```python
from build123d import *

# Parameters (mm, degrees)
SKETCH_R      = 1.75
EXTRUDE_DEPTH = 1


with BuildPart() as part:
    # Sketch → Extrude (new body)
    with BuildSketch(Plane.XY):
        with BuildLine():
            Line((65.264214, 54.65), (67.4, 52.514214))
            Line((67.4, 52.514214), (67.4, 41.014214))
            Line((67.4, 41.014214), (69.95, 38.464214))
            Line((69.95, 38.464214), (69.95, 4.685786))
            Line((69.95, 4.685786), (67.4, 2.135786))
            Line((67.4, 2.135786), (67.4, 1))
            ThreePointArc((65.4, -1), (66.814214, -0.414214), (67.4, 1))
            Line((65.4, -1), (1, -1))
            ThreePointArc((-1, 1), (-0.414214, -0.414214), (1, -1))
            Line((-1, 1), (-1, 52.65))
            ThreePointArc((1, 54.65), (-0.414214, 54.064214), (-1, 52.65))
            Line((1, 54.65), (65.264214, 54.65))
        make_face()
        with Locations((14.05247, 2.556984)):
            Circle(SKETCH_R, mode=Mode.SUBTRACT)
        with Locations((66.413926, 7.668398)):
            Circle(SKETCH_R, mode=Mode.SUBTRACT)
        with Locations((66.409951, 35.749834)):
            Circle(SKETCH_R, mode=Mode.SUBTRACT)
        with Locations((15.334135, 51.082933)):
            Circle(SKETCH_R, mode=Mode.SUBTRACT)
    extrude(amount=EXTRUDE_DEPTH)


solid = part.part
```
Source: CAD feature listing. Evaluate the final solid. Frame: model axes, mm. Give positions to 0.01 mm unless a question says otherwise; leave off trailing zeros. Loops run counter-clockwise (first coordinate to the right, second up) from the corner with the lowest first, then second, coordinate; pieces in that order, holes last. Notation, with made-up numbers: (-6, 68.25) -> (41, 68.25) arc R32 ccw to (41, 100.25) -> close; hole circle Ø7 at (-39.5, 21.25). An arc over 180 degrees is marked (long way). Use a Markdown table: item, result. Add a question column.
(1) Section query B-B (y = 42). Output: boundary loops of the cut face in (x, z), then the cut area to 3 significant figures.
(2) Ray query, line 1 (Y direction, x = 15, z = 0.45); line 2 (Y direction, x = 65, z = 0.55); line 3 (X direction, y = 43, z = 0.5). Return the intervals inside material, ascending.
(3) Pull-direction query (X, two-part tool) for faces 1 (the face through (-0.43, -0.4, 0.49)), 2 (the face through (68.693, 3.429, 0.493)), 3 (the face through (35, 27, 0)), 4 (the face through (68.083, 8.194, 0.493)); classes: +X half, -X half, draft (parallel to the pull), parting line (faces both ways), or undercut.
(4) Section query A-A (z = 0.8). Output: boundary loops of the cut face in (x, y), then the cut area to 3 significant figures.
Checked values:
| question | item | result |
|---|---|---|
| 1 | outline | (-1, 0) -> (67.4, 0) -> (67.4, 1) -> (-1, 1) -> close |
| 1 | area | 68.4 mm^2 |
| 2 | line 1 | -1 to 1.09, 4.03 to 49.37, 52.8 to 54.65 |
| 2 | line 2 | -1 to 6.64, 8.7 to 34.71, 36.79 to 54.65 |
| 2 | line 3 | -1 to 67.4 |
| 3 | face 1 | -X half |
| 3 | face 2 | +X half |
| 3 | face 3 | draft |
| 3 | face 4 | undercut |
| 4 | outline | (-1, 1) arc R2 ccw to (1, -1) -> (65.4, -1) arc R2 ccw to (67.4, 1) -> (67.4, 2.14) -> (69.95, 4.69) -> (69.95, 38.46) -> (67.4, 41.01) -> (67.4, 52.51) -> (65.26, 54.65) -> (1, 54.65) arc R2 ccw to (-1, 52.65) -> close; hole circle Ø3.5 at (14.05, 2.56); hole circle Ø3.5 at (15.33, 51.08); hole circle Ø3.5 at (66.41, 7.67); hole circle Ø3.5 at (66.41, 35.75) |
| 4 | area | 3,860 mm^2 |
